The listing builds one solid part. Answer for the finished solid, in the listing's coordinates (mm). Face numbers are marked on the shaded views. A direction names the side the tool comes from. Coordinates: 2 decimals unless noted, no trailing zeros. Order: outer loops, then holes, each group sorted by start corner. A loop starts at its lowest first (then second) coordinate and runs counter-clockwise, first axis right, second up.
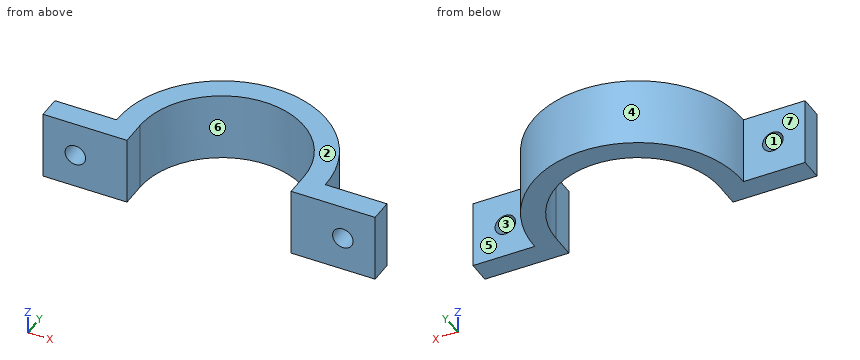
```python
from build123d import *

# Parameters (mm, degrees)
BOSS_EXTRUDE1_DEPTH     = 15
SKETCH5_R               = 2.25
CUT_EXTRUDE1_DEPTH      = 24.3125
CUT_EXTRUDE1_DEPTH_BACK = 6


with BuildPart() as part:
    # Sketch3 → Boss-Extrude1 (new body)
    with BuildSketch(Plane.XY):
        with BuildLine():
            Line((18, 0), (18, -5.4125))
            Line((18, -5.4125), (36.4334, -5.4125))
            Line((36.4334, -5.4125), (36.4334, -0.4125))
            Line((36.4334, -0.4125), (22.896284497, -0.4125))
            ThreePointArc((22.896284497, -0.4125), (0, 22.9), (-22.896284497, -0.4125))
            Line((-22.896284497, -0.4125), (-36.4334, -0.4125))
            Line((-36.4334, -0.4125), (-36.4334, -5.4125))
            Line((-36.4334, -5.4125), (-18, -5.4125))
            Line((-18, -5.4125), (-18, 0))
            ThreePointArc((-18, 0), (0, 18), (18, 0))
        make_face()
    extrude(amount=BOSS_EXTRUDE1_DEPTH)

    # Sketch5 → Cut-Extrude1 (cut, two sides)
    with BuildSketch(Plane(origin=(0, -0.4125, 0), x_dir=(1, 0, 0), z_dir=(0, 1, 0))) as cut_extrude1_sk:
        with Locations((-29.3423, -7.5)):
            Circle(SKETCH5_R)
        with Locations((29.3423, -7.5)):
            Circle(SKETCH5_R)
    extrude(amount=CUT_EXTRUDE1_DEPTH, mode=Mode.SUBTRACT)
    extrude(cut_extrude1_sk.sketch, amount=-CUT_EXTRUDE1_DEPTH_BACK, mode=Mode.SUBTRACT)


solid = part.part
```
(1) For the marked faces 5, 6 and 7, determine the directions among +Z, -Z, +X, -X, +Y, -Y from which every point of the face is accessible in a straight line to the end or side of a thin tool.
(2) Consider line 1 (X direction, y = -1.6, z = 7.5); line 2 (X direction, y = -1.25, z = 13); line 3 (X direction, y = 0, z = 13). Determine where each line is inside the solid, lowest interval first.
(3) Find section D-D (x = 0). Write down the section's boundary in (y, z), and give its area (3 significant figures).
(4) Each of these flat-tipped pins is pushed along its axis until it touches: pin 1 Ø3 at (x, z) = (9.5, 2.5) entering from -Y; pin 2 Ø3 at (y, z) = (16.5, 2.5) entering from -X; pin 3 Ø7 at (x, z) = (-29.34, 7.5) entering from +Y. Where does it stop, or does it pass through?
(5) Find section C-C (y = 11). Write down the section's boundary in (x, z), and give its area (3 significant figures).
(6) The mould has two halves that part along X. Classify the marked faces 1, 2, 3 and 4: released by +X, released by -X, zero draft, split by the parting line, or undercut.
Findings below:
1. face 5: +Z, -Z, +X, +Y
1. face 6: +Z, -Z, -Y
1. face 7: +Z, -Z, -X, +Y
2. line 1: x = -36.43 to -31.59, -27.09 to -18, 18 to 27.09, 31.59 to 36.43
2. line 2: x = -36.43 to -18, 18 to 36.43
2. line 3: x = -22.9 to -18, 18 to 22.9
3. outline: (18, 0) - (22.9, 0) - (22.9, 15) - (18, 15) - close
3. area: 73.5 mm2
4. pin 1: stops at y = 14.25
4. pin 2: stops at x = -17.3
4. pin 3: stops at y = -0.41
5. outline: (-20.09, 0) - (-14.25, 0) - (-14.25, 15) - (-20.09, 15) - close; (14.25, 0) - (20.09, 0) - (20.09, 15) - (14.25, 15) - close
5. area: 175 mm2
6. face 1: undercut
6. face 2: zero draft
6. face 3: undercut
6. face 4: split by the parting line
